Design review of the part built by this model. Coordinates are the model's own, in mm. Coordinates: 2 decimals unless noted, no trailing zeros. Loops run counter-clockwise (first coordinate to the right, second up) from the corner with the lowest first, then second, coordinate; pieces in that order, holes last.
from build123d import *

# Parameters (mm, degrees)
SKETCH1_W               = 19.05
SKETCH1_H               = 50.8
BOSS_EXTRUDE1_DEPTH     = 1.5875
M4_CLEARANCE_HOLE1_D    = 4.5
SKETCH4_W               = 19.05
SKETCH4_H               = 7.62
BOSS_EXTRUDE2_DEPTH     = 1.5875
FILLET1_R               = 2.54
CUT_EXTRUDE1_DEPTH      = 35.40299669
CUT_EXTRUDE1_DEPTH_BACK = 35.40299669


with BuildPart() as part:
    # Sketch1 → Boss-Extrude1 (new body)
    with BuildSketch(Plane.XY):
        Rectangle(SKETCH1_W, SKETCH1_H)
    extrude(amount=BOSS_EXTRUDE1_DEPTH)

    # M4 Clearance Hole1 (through all)
    with Locations(Plane.XY.offset(1.5875)):
        with Locations((0, 17.6276), (0, -17.6276)):
            Hole(M4_CLEARANCE_HOLE1_D / 2)

    # Sketch4 → Boss-Extrude2 (add)
    with BuildSketch(Plane.XY.offset(1.5875)):
        with Locations((0, -29.21)):
            Rectangle(SKETCH4_W, SKETCH4_H)
    extrude(amount=-BOSS_EXTRUDE2_DEPTH)

    # Fillet1
    fillet1_edges = [part.edges().sort_by_distance(p)[0] for p in [
        (-9.525, 25.4, 0.79375),
        (9.525, 25.4, 0.79375),
    ]]
    fillet(fillet1_edges, radius=FILLET1_R)

    # Sketch5 → Cut-Extrude1 (cut, two sides: drawn at the far end of the back side and taken through both)
    with BuildSketch(Plane.XY.offset(1.5875).offset(-CUT_EXTRUDE1_DEPTH_BACK)):
        Polygon((9.525, -29.845), (-9.525, -33.02), (9.525, -33.02), align=None)
    extrude(amount=CUT_EXTRUDE1_DEPTH + CUT_EXTRUDE1_DEPTH_BACK, mode=Mode.SUBTRACT)


solid = part.part
Q1. Take a section at A-A, the plane x = 0. Write out the cut boundary in (y, z), then the cut area to 3 significant figures.
Q2. Take a section at C-C, the plane x = 3.5. Write out the cut boundary in (y, z).
Q3. Take a section at B-B, the plane z = 1.3. Write out the cut boundary in (x, y) (3 decimals).
Q4. For line 1 (Y direction, x = 0, z = 1.1); line 2 (Y direction, x = -1.5, z = 1.15); line 3 (X direction, y = -16, z = 0.8) (3 decimals), list the stretches that pass through material, from the lowest coordinate up.
Q5. The part is to be moulded in two halves that separate along X. For faces 1 (the cylindrical face through (8.801, 24.636, 0.805)), 2 (the flat face through (0, 25.4, 1)), 3 (the cylindrical face through (-1.21, -15.73, 0.78)), say which applies: pulls with the +X half, pulls with the -X half, needs draft (parallel to the pull), parting line crosses it, or undercut.
Q6. Clearance check with a flat-ended pin moving along its axis: pin 1 Ø3.5 at (x, y) = (0, 17.63) entering from -Z. State where the tip first meets the part, or that it passes through.
Entries:
1. outline: (-31.43, 0) - (-19.88, 0) - (-19.88, 1.59) - (-31.43, 1.59) - close; (-15.38, 0) - (15.38, 0) - (15.38, 1.59) - (-15.38, 1.59) - close; (19.88, 0) - (25.4, 0) - (25.4, 1.59) - (19.88, 1.59) - close
1. area: 75.9 mm2
2. outline: (-30.85, 0) - (25.4, 0) - (25.4, 1.59) - (-30.85, 1.59) - close
3. outline: (-9.525, -33.02) - (9.525, -29.845) - (9.525, 22.86) arc R2.54 ccw to (6.985, 25.4) - (-6.985, 25.4) arc R2.54 ccw to (-9.525, 22.86) - close; hole circle Ø4.5 at (0, -17.628); hole circle Ø4.5 at (0, 17.628)
4. line 1: y = -31.43 to -19.88, -15.38 to 15.38, 19.88 to 25.4
4. line 2: y = -31.68 to -19.3, -15.95 to 15.95, 19.3 to 25.4
4. line 3: x = -9.525 to -1.554, 1.554 to 9.525
5. face 1: pulls with the +X half
5. face 2: needs draft
5. face 3: undercut
6. pin 1: passes through
